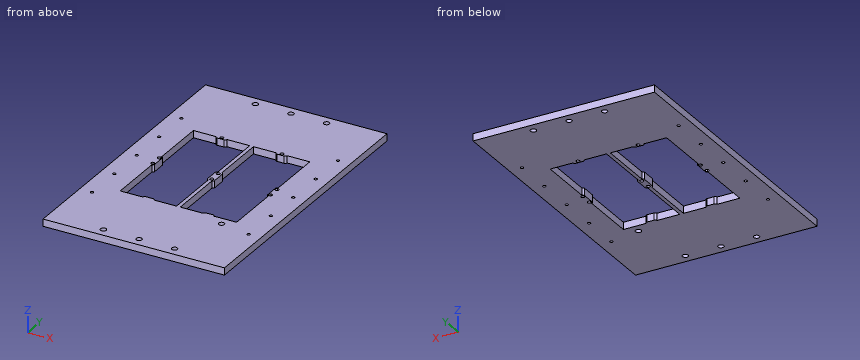
from build123d import *

# Parameters (mm, degrees)
F0_W     = 255
F0_H     = 400
F0_R     = 2.1
F0_R_2   = 4
F0_R_3   = 2.5
F1_DEPTH = 10
F2_R     = 4
F3_DEPTH = 10.001


with BuildPart() as f1:
    # F0 (on Top) → F1 (new body)
    with BuildSketch(Plane.XY):
        Rectangle(F0_W, F0_H)
        with Locations((-110, -110)):
            Circle(F0_R, mode=Mode.SUBTRACT)
        with Locations((-50, -187)):
            Circle(F0_R_2, mode=Mode.SUBTRACT)
        with Locations((-110, -55)):
            Circle(F0_R, mode=Mode.SUBTRACT)
        with Locations((0, -187)):
            Circle(F0_R_2, mode=Mode.SUBTRACT)
        with Locations((50, -187)):
            Circle(F0_R_2, mode=Mode.SUBTRACT)
        with Locations((110, -110)):
            Circle(F0_R, mode=Mode.SUBTRACT)
        with Locations((0, -8)):
            Circle(F0_R_3, mode=Mode.SUBTRACT)
        with Locations((110, -55)):
            Circle(F0_R, mode=Mode.SUBTRACT)
        with Locations((-110, 0)):
            Circle(F0_R, mode=Mode.SUBTRACT)
        with Locations((-110, 55)):
            Circle(F0_R, mode=Mode.SUBTRACT)
        with BuildLine():
            Line((-34.7, 90.1), (-2.6, 90.1))
            Line((-2.6, 90.1), (-2.6, 11.8))
            Line((-2.6, 11.8), (-2.6, -11.8))
            Line((-2.6, -11.8), (-2.6, -90.1))
            Line((-2.6, -90.1), (-34.7, -90.1))
            Line((-34.7, -90.1), (-49.7, -90.1))
            Line((-49.7, -90.1), (-81.8, -90.1))
            Line((-81.8, -90.1), (-81.8, -11.8))
            Line((-81.8, -11.8), (-81.8, -10.291288))
            ThreePointArc((-81.8, -10.291288), (-85.3, -8), (-81.8, -5.708712))
            Line((-81.8, -5.708712), (-81.8, 5.708712))
            ThreePointArc((-81.8, 5.708712), (-85.3, 8), (-81.8, 10.291288))
            Line((-81.8, 10.291288), (-81.8, 11.8))
            Line((-81.8, 11.8), (-81.8, 90.1))
            Line((-81.8, 90.1), (-49.7, 90.1))
            Line((-49.7, 90.1), (-44.491288, 90.1))
            ThreePointArc((-44.491288, 90.1), (-42.710774, 93.547266), (-39.7, 91.1))
            ThreePointArc((-39.7, 91.1), (-39.752734, 90.589226), (-39.908712, 90.1))
            Line((-39.908712, 90.1), (-34.7, 90.1))
        make_face(mode=Mode.SUBTRACT)
        with Locations((-110, 110)):
            Circle(F0_R, mode=Mode.SUBTRACT)
        with Locations((-50, 187)):
            Circle(F0_R_2, mode=Mode.SUBTRACT)
        with Locations((0, 8)):
            Circle(F0_R_3, mode=Mode.SUBTRACT)
        with BuildLine():
            Line((2.6, 11.8), (2.6, 90.1))
            Line((2.6, 90.1), (34.7, 90.1))
            Line((34.7, 90.1), (39.908712, 90.1))
            ThreePointArc((39.908712, 90.1), (41.689226, 93.547266), (44.7, 91.1))
            ThreePointArc((44.7, 91.1), (44.647266, 90.589226), (44.491288, 90.1))
            Line((44.491288, 90.1), (49.7, 90.1))
            Line((49.7, 90.1), (81.8, 90.1))
            Line((81.8, 90.1), (81.8, 11.8))
            Line((81.8, 11.8), (81.8, 10.291288))
            ThreePointArc((81.8, 10.291288), (84.169306, 10.09165), (85.3, 8))
            ThreePointArc((85.3, 8), (84.169306, 5.90835), (81.8, 5.708712))
            Line((81.8, 5.708712), (81.8, -5.708712))
            ThreePointArc((81.8, -5.708712), (84.169306, -5.90835), (85.3, -8))
            ThreePointArc((85.3, -8), (84.169306, -10.09165), (81.8, -10.291288))
            Line((81.8, -10.291288), (81.8, -11.8))
            Line((81.8, -11.8), (81.8, -90.1))
            Line((81.8, -90.1), (49.7, -90.1))
            Line((49.7, -90.1), (34.7, -90.1))
            Line((34.7, -90.1), (2.6, -90.1))
            Line((2.6, -90.1), (2.6, -11.8))
            Line((2.6, -11.8), (2.6, 11.8))
        make_face(mode=Mode.SUBTRACT)
        with Locations((110, 0)):
            Circle(F0_R, mode=Mode.SUBTRACT)
        with Locations((110, 55)):
            Circle(F0_R, mode=Mode.SUBTRACT)
        with Locations((0, 187)):
            Circle(F0_R_2, mode=Mode.SUBTRACT)
        with Locations((50, 187)):
            Circle(F0_R_2, mode=Mode.SUBTRACT)
        with Locations((110, 110)):
            Circle(F0_R, mode=Mode.SUBTRACT)
        with BuildLine():
            Line((81.8, 10.291288), (81.8, 11.8))
            ThreePointArc((81.8, 11.8), (80.3, 11.3), (79.4, 10))
            Line((79.4, 10), (79.4, 0))
            Line((79.4, 0), (79.4, -10))
            ThreePointArc((79.4, -10), (80.3, -11.3), (81.8, -11.8))
            Line((81.8, -11.8), (81.8, -10.291288))
            ThreePointArc((81.8, -10.291288), (80.3, -8), (81.8, -5.708712))
            Line((81.8, -5.708712), (81.8, 5.708712))
            ThreePointArc((81.8, 5.708712), (80.3, 8), (81.8, 10.291288))
        make_face()
        with BuildLine():
            Line((39.908712, 90.1), (34.7, 90.1))
            ThreePointArc((34.7, 90.1), (35.432233, 88.332233), (37.2, 87.6))
            Line((37.2, 87.6), (42.2, 87.6))
            Line((42.2, 87.6), (47.2, 87.6))
            ThreePointArc((47.2, 87.6), (48.967767, 88.332233), (49.7, 90.1))
            Line((49.7, 90.1), (44.491288, 90.1))
            ThreePointArc((44.491288, 90.1), (42.2, 88.6), (39.908712, 90.1))
        make_face()
        with BuildLine():
            ThreePointArc((37.2, -87.6), (35.432233, -88.332233), (34.7, -90.1))
            Line((34.7, -90.1), (49.7, -90.1))
            ThreePointArc((49.7, -90.1), (48.967767, -88.332233), (47.2, -87.6))
            Line((47.2, -87.6), (42.2, -87.6))
            Line((42.2, -87.6), (37.2, -87.6))
        make_face()
        with BuildLine():
            ThreePointArc((5, 10), (4.1, 11.3), (2.6, 11.8))
            Line((2.6, 11.8), (2.6, -11.8))
            ThreePointArc((2.6, -11.8), (4.1, -11.3), (5, -10))
            Line((5, -10), (5, 0))
            Line((5, 0), (5, 10))
        make_face()
        with BuildLine():
            Line((-2.6, -11.8), (-2.6, 11.8))
            ThreePointArc((-2.6, 11.8), (-4.1, 11.3), (-5, 10))
            Line((-5, 10), (-5, 0))
            Line((-5, 0), (-5, -10))
            ThreePointArc((-5, -10), (-4.1, -11.3), (-2.6, -11.8))
        make_face()
        with BuildLine():
            ThreePointArc((-79.4, 10), (-80.3, 11.3), (-81.8, 11.8))
            Line((-81.8, 11.8), (-81.8, 10.291288))
            ThreePointArc((-81.8, 10.291288), (-80.70835, 9.369306), (-80.3, 8))
            ThreePointArc((-80.3, 8), (-80.70835, 6.630694), (-81.8, 5.708712))
            Line((-81.8, 5.708712), (-81.8, -5.708712))
            ThreePointArc((-81.8, -5.708712), (-80.70835, -6.630694), (-80.3, -8))
            ThreePointArc((-80.3, -8), (-80.70835, -9.369306), (-81.8, -10.291288))
            Line((-81.8, -10.291288), (-81.8, -11.8))
            ThreePointArc((-81.8, -11.8), (-80.3, -11.3), (-79.4, -10))
            Line((-79.4, -10), (-79.4, 0))
            Line((-79.4, 0), (-79.4, 10))
        make_face()
        with BuildLine():
            ThreePointArc((-37.2, 87.6), (-35.432233, 88.332233), (-34.7, 90.1))
            Line((-34.7, 90.1), (-39.908712, 90.1))
            ThreePointArc((-39.908712, 90.1), (-42.2, 88.6), (-44.491288, 90.1))
            Line((-44.491288, 90.1), (-49.7, 90.1))
            ThreePointArc((-49.7, 90.1), (-48.967767, 88.332233), (-47.2, 87.6))
            Line((-47.2, 87.6), (-42.2, 87.6))
            Line((-42.2, 87.6), (-37.2, 87.6))
        make_face()
        with BuildLine():
            Line((-49.7, -90.1), (-34.7, -90.1))
            ThreePointArc((-34.7, -90.1), (-35.432233, -88.332233), (-37.2, -87.6))
            Line((-37.2, -87.6), (-42.2, -87.6))
            Line((-42.2, -87.6), (-47.2, -87.6))
            ThreePointArc((-47.2, -87.6), (-48.967767, -88.332233), (-49.7, -90.1))
        make_face()
    extrude(amount=F1_DEPTH)

    # F2 (on face) → F3 (cut, through all)
    with BuildSketch(Plane.XY.offset(10)):
        with Locations((67.8, -102.6)):
            Circle(F2_R)
    extrude(amount=-F3_DEPTH, mode=Mode.SUBTRACT)


solid = f1.part
The listing builds one solid part. Answer for the finished solid, in the listing's coordinates (mm). Give positions to 0.01 mm unless a question says otherwise; leave off trailing zeros. Order: outer loops, then holes, each group sorted by start corner. A loop starts at its lowest first (then second) coordinate and runs counter-clockwise, first axis right, second up. Notation, with made-up numbers: (45, -33.75) - (97, -33.75) arc R21 cw to (97, -4.75) - close; hole circle Ø5 at (11.25, 32.5). An arc over 180 degrees is marked (long way). One line per item, written item: value. Start each with the question number.
1) Find the intervals of material crossed by L1, parallel to Y at x = 110, z = 4.5; L2, parallel to Y at x = -50, z = 7.5; L3, parallel to X at y = 74, z = 2.5, in increasing order.
2) A cutting plane is placed at D-D on z = 4.75. State how many separate pieces and enclosed holes the cut face has, then the cut area to 3 significant figures.
3) A cutting plane is placed at B-B on y = 187. Give the vertices of the cut face in (x, z).
4) A cutting plane is placed at A-A on x = -13. Give the vertices of the cut face in (y, z), then the cut area to 3 significant figures.
5) A cutting plane is placed at C-C on x = 67.8. Give the vertices of the cut face in (y, z).
Answer sheet:
1. L1: y = -200 to -112.1, -107.9 to -57.1, -52.9 to -2.1, 2.1 to 52.9, 57.1 to 107.9, 112.1 to 200
1. L2: y = -200 to -191, -183 to -90.1, 90.1 to 183, 191 to 200
1. L3: x = -127.5 to -81.8, -2.6 to 2.6, 81.8 to 127.5
2. separate pieces: 1
2. enclosed holes: 27
2. area: 73,200 mm2
3. outline: (-127.5, 0) - (-54, 0) - (-54, 10) - (-127.5, 10) - close; (-46, 0) - (-4, 0) - (-4, 10) - (-46, 10) - close; (4, 0) - (46, 0) - (46, 10) - (4, 10) - close; (54, 0) - (127.5, 0) - (127.5, 10) - (54, 10) - close
4. outline: (-200, 0) - (-90.1, 0) - (-90.1, 10) - (-200, 10) - close; (90.1, 0) - (200, 0) - (200, 10) - (90.1, 10) - close
4. area: 2,200 mm2
5. outline: (-200, 0) - (-106.6, 0) - (-106.6, 10) - (-200, 10) - close; (-98.6, 0) - (-90.1, 0) - (-90.1, 10) - (-98.6, 10) - close; (90.1, 0) - (200, 0) - (200, 10) - (90.1, 10) - close
